from build123d import *

# Parameters (mm, degrees)
SKETCH2_W          = 8
SKETCH2_H          = 20
CUT_EXTRUDE1_DEPTH = 313.594035852
SKETCH3_R          = 12.5
CUT_EXTRUDE2_DEPTH = 281.606541709


with BuildPart() as part:
    # Sketch1 → Revolve1 (revolve)
    with BuildSketch(Plane(origin=(0, 0, 0), x_dir=(1, 0, 0), z_dir=(0, 1, 0)), mode=Mode.PRIVATE) as revolve1_sk:
        Polygon((-13.77173913, 35), (128.22826087, 35), (128.22826087, 80), (23.22826087, 80), (23.22826087, 85), (-16.77173913, 85), (-16.77173913, 143), (8.22826087, 143), (8.22826087, 169.875), (-66.77173913, 169.875), (-66.77173913, 90), (-71.77173913, 90), (-71.77173913, 60), (-13.77173913, 60), align=None)
    revolve(revolve1_sk.sketch.rotate(Axis((-159.75, 0, 0), (1, 0, 0)), 180), axis=Axis((-159.75, 0, 0), (1, 0, 0)))

    # Sketch2 → Cut-Extrude1 (cut, through all)
    with BuildSketch(Plane(origin=(128.22826087, 0, 0), x_dir=(0, 0, -1), z_dir=(1, 0, 0))):
        with Locations((37.541019662, 0)):
            Rectangle(SKETCH2_W, SKETCH2_H)
    extrude(amount=-CUT_EXTRUDE1_DEPTH, mode=Mode.SUBTRACT)

    # Sketch3 → Cut-Extrude2 (cut, through all)
    with BuildSketch(Plane(origin=(-16.77173913, 0, 0), x_dir=(0, 0, -1), z_dir=(1, 0, 0))):
        with Locations((0, 108.805263326)):
            Circle(SKETCH3_R)
        with Locations((94.228122106, 54.402631663)):
            Circle(SKETCH3_R)
        with Locations((94.228122106, -54.402631663)):
            Circle(SKETCH3_R)
        with Locations((0, -108.805263326)):
            Circle(SKETCH3_R)
        with Locations((-94.228122106, -54.402631663)):
            Circle(SKETCH3_R)
        with Locations((-94.228122106, 54.402631663)):
            Circle(SKETCH3_R)
    extrude(amount=-CUT_EXTRUDE2_DEPTH, mode=Mode.SUBTRACT)


solid = part.part
Verification items for the finished model (mm, model axes). A direction names the side the tool comes from. Coordinates: 2 decimals unless noted, no trailing zeros. Order: outer loops, then holes, each group sorted by start corner. A loop starts at its lowest first (then second) coordinate and runs counter-clockwise, first axis right, second up. Notation, with made-up numbers: (46.5, 61.5) -> (79.5, 61.5) arc R16 ccw to (79.5, 71.5) -> close; hole circle Ø1 at (-23, 53.25). An arc over 180 degrees is marked (long way). Use CSV: the item, a comma, the result in double quotes. Start each with the question number.
Q1. Tool access check on faces 1 (the cylindrical face through (-4.097, -96.646, -105.397)), 2 (the flat face through (58, 0, -41.541)), 3 (the flat face through (-13.772, 26, 26)), 4 (the flat face through (128.228, 17, -34)), 5 (the flat face through (-71.772, 59, 19)). Record the directions out of +Z, -Z, +X, -X, +Y, -Y that give a thin tool (end or side, any length) a straight path to the whole face; none if there is none.
Q2. Section check A-A, the plane y = 0. Record the cut outline in (x, z) (3 decimals).
Q3. Thickness scan on line 1 along Y through (x, z) = (-31, 0) (3 decimals); line 2 along Y through (x, z) = (-4.5, 13.5); line 3 along Z through (x, y) = (-5, -68.5). Record the ranges inside material, lowest first.
Q4. Section check D-D, the plane z = 0. Give the number of separate pieces and of enclosed holes in the cut face, and give its area (3 significant figures).
Q5. Section check C-C, the plane x = 97. Record the cut outline in (y, z).
Q6. Depth check by flat-ended pin: P1, Ø12, axis at x = 12.5, z = 115, coming from the -Y side; P2, Ø1, axis at y = -130, z = -100.5, coming from the -X side; P3, Ø6, axis at x = 78.5, y = -39, coming from the +Z side. Enter the tip coordinate at first touch or a pass-through.
Q7. Draft check along Z on faces 6 (the cylindrical face through (-41.422, -59.19, -105.775)), 7 (the cylindrical face through (74.993, -3.517, -79.923)), 8 (the flat face through (-16.772, 62, -62)), 9 (the flat face through (-66.772, 73, 73)). Enter one of: +Z half, -Z half, draft (parallel to the pull), parting line (faces both ways), or undercut.
Q8. Section check B-B, the plane x = -43.5. Record the cut outline in (y, z) (3 decimals).
Returned:
1,face 1,"+X"
1,face 2,"+X, -X"
1,face 3,"-X"
1,face 4,"+Z, -Z, +X, +Y, -Y"
1,face 5,"+Z, -Z, -X, +Y, -Y"
2,outline,"(-71.772, -90) -> (-66.772, -90) -> (-66.772, -169.875) -> (8.228, -169.875) -> (8.228, -143) -> (-16.772, -143) -> (-16.772, -85) -> (23.228, -85) -> (23.228, -80) -> (128.228, -80) -> (128.228, -41.541) -> (-13.772, -41.541) -> (-13.772, -60) -> (-71.772, -60) -> close; (-71.772, 60) -> (-13.772, 60) -> (-13.772, 35) -> (128.228, 35) -> (128.228, 80) -> (23.228, 80) -> (23.228, 85) -> (-16.772, 85) -> (-16.772, 143) -> (8.228, 143) -> (8.228, 169.875) -> (-66.772, 169.875) -> (-66.772, 90) -> (-71.772, 90) -> close"
3,line 1,"y = -169.875 to -121.305, -96.305 to -60, 60 to 96.305, 121.305 to 169.875"
3,line 2,"y = -169.34 to -142.36, -83.92 to -32.29, 32.29 to 83.92, 142.36 to 169.34"
3,line 3,"z = -155.45 to -125.53, -50.33 to 50.33, 125.53 to 155.45"
4,separate pieces,"4"
4,enclosed holes,"0"
4,area,"23,400 mm^2"
5,outline,"circle Ø160 at (0, 0); hole (-10, -41.54) -> (10, -41.54) -> (10, -33.54) arc R35 ccw (long way) to (-10, -33.54) -> close"
6,P1,"stops at y = -128.78"
6,P2,"stops at x = -66.77"
6,P3,"stops at z = 71.44"
7,face 6,"undercut"
7,face 7,"parting line"
7,face 8,"undercut"
7,face 9,"draft"
8,outline,"circle Ø339.75 at (0, 0); hole circle Ø25 at (-108.805, 0); hole circle Ø25 at (-54.403, -94.228); hole circle Ø25 at (-54.403, 94.228); hole circle Ø120 at (0, 0); hole circle Ø25 at (54.403, -94.228); hole circle Ø25 at (54.403, 94.228); hole circle Ø25 at (108.805, 0)"
